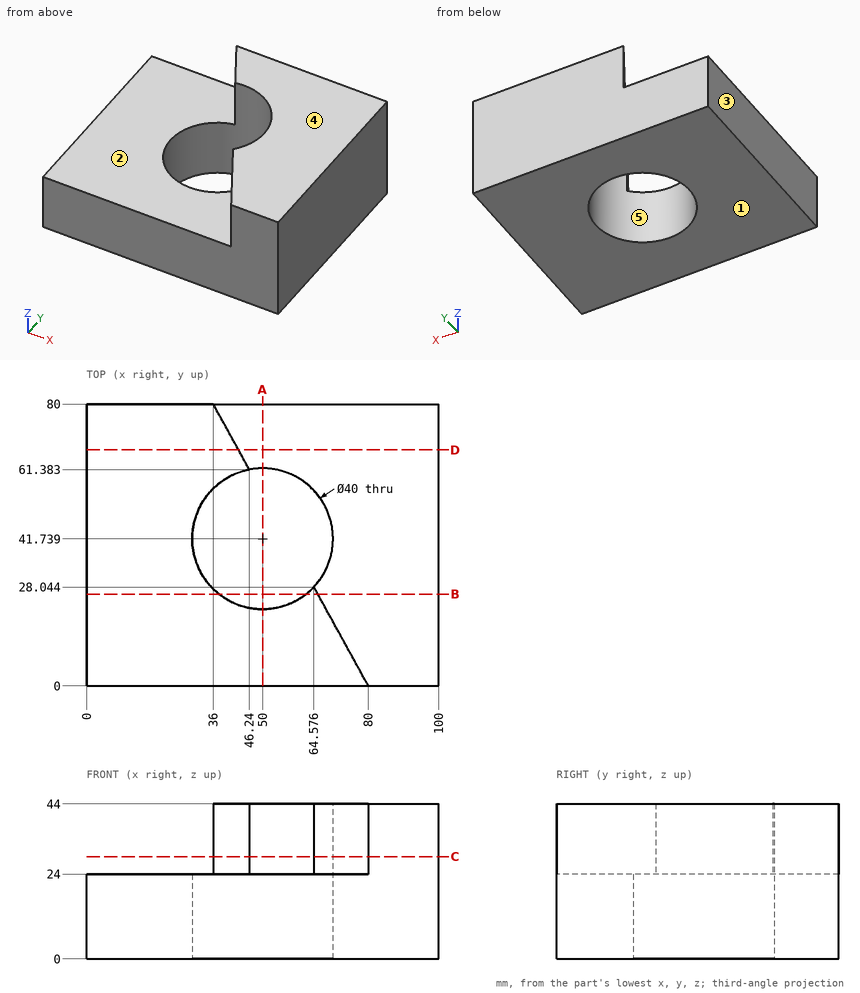
Study the drawing (mm; zero at the part's minimum x, y, z) and answer. A direction names the side the tool comes from. Coordinates: 2 decimals unless noted, no trailing zeros. Loops run counter-clockwise (first coordinate to the right, second up) from the corner with the lowest first, then second, coordinate; pieces in that order, holes last. Notation, with made-up numbers: (-3, 4) -> (50, 4) arc R34 cw to (50, 35) -> close; hole circle Ø9 at (49.25, -37). An arc over 180 degrees is marked (long way). Write item = value, one per line. Start each with the question number.
1) The part is cut by section B-B, the plane y = 26. Determine the outline of the cut face in (x, z).
2) For the marked faces 1 and 2, determine the directions among +Z, -Z, +X, -X, +Y, -Y from which every point of the face is accessible in a straight line to the end or side of a thin tool.
3) The part is cut by section D-D, the plane y = 67. Determine the outline of the cut face in (x, z).
4) Find the intervals of material crossed by L1, parallel to Y at x = 50, z = 12; L2, parallel to Z at x = 67.5, y = 11; L3, parallel to X at y = 47.5, z = 15.5, in increasing order. Write a range as from..to.
5) The mould has two halves that part along X. Classify the marked faces 3, 4 and 5: pulls with the +X half, pulls with the -X half, needs draft (parallel to the pull), parting line crosses it, or undercut.
6) The part is cut by section C-C, the plane z = 29. Determine the outline of the cut face in (x, y) (1 decimal).
7) The part is cut by section A-A, the plane x = 50. Determine the outline of the cut face in (y, z), plus the area to 3 significant figures.
8) Given P1, Ø5, axis at y = 61.5, z = 18, coming from the -X side; P2, Ø6, axis at x = 33, y = 14, coming from the +Z side; P3, Ø8, axis at y = 23, z = 31.5, coming from the -X side; P4, Ø12, axis at y = 38, z = 34, coming from the -X side, each flat-ended and moving along its own axis, determine where each tip first touches the part or whether it passes through.
Result:
q1.outline = (0, 0) -> (37.66, 0) -> (37.66, 24) -> (0, 24) -> close; (62.34, 0) -> (100, 0) -> (100, 44) -> (65.7, 44) -> (65.7, 24) -> (62.34, 24) -> close
q2.face_1 = -Z, +X, -X, +Y, -Y
q2.face_2 = +Z, -X, -Y
q3.outline = (0, 0) -> (100, 0) -> (100, 44) -> (43.15, 44) -> (43.15, 24) -> (0, 24) -> close
q4.L1 = 0..21.74, 61.74..80
q4.L2 = 0..24
q4.L3 = 0..30.85, 69.15..100
q5.face_3 = pulls with the -X half
q5.face_4 = needs draft
q5.face_5 = undercut
q6.outline = (36, 80) -> (46.2, 61.4) arc R20 cw to (64.6, 28) -> (80, 0) -> (100, 0) -> (100, 80) -> close
q7.outline = (0, 0) -> (21.74, 0) -> (21.74, 24) -> (0, 24) -> close; (61.74, 0) -> (80, 0) -> (80, 44) -> (61.74, 44) -> close
q7.area = 1,330 mm²
q8.P1 = 0
q8.P2 = 24
q8.P3 = 65.15
q8.P4 = 67.47
